Print and shaded views of the part. All mm, measured from the part's lowest x, y and z. Round coordinates to 2 decimals unless told otherwise and drop trailing zeros. Order: outer loops, then holes, each group sorted by start corner. A loop starts at its lowest first (then second) coordinate and runs counter-clockwise, first axis right, second up. Notation, with made-up numbers: (33, 35.5) - (46, 35.5) arc R20 cw to (46, 46.5) - close; hole circle Ø6 at (-34, 37). An arc over 180 degrees is marked (long way). Return JSON: item names as keys, results as strings. Group by question number.
Item 1: Probe probe 1 along Z at (x, y) = (2.25, 1); probe 2 along Z at (x, y) = (6.5, 6.75); probe 3 along X at (y, z) = (3.75, 46.5). List the from-to ranges inside material, lowest first.
Item 2: Saw through at A-A on z = 8.5. List the corners of the cut face in (x, y), and give its area (3 significant figures).
Item 3: Drop flat-ended pins along their axis: pin 1 (3 mm diameter, centred on y = 6, z = 15, fed in from +X); pin 2 (1.5 mm diameter, centred on x = 6.5, z = 34.5, fed in from -Y); pin 3 (4 mm diameter, centred on x = 7, z = 24, fed in from +Y). Give the stop position or say it passes through.
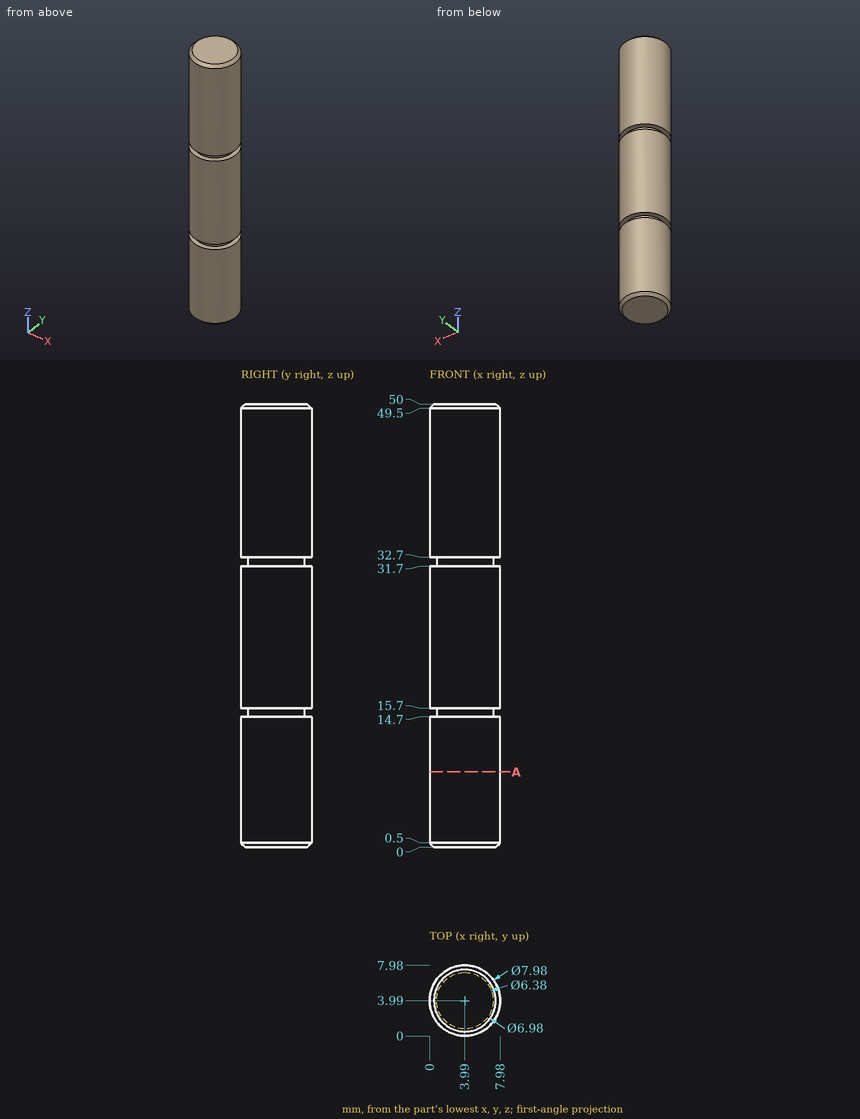
Filled in:
{
 "1": {"probe 1": "z = 0 to 14.7, 15.7 to 31.7, 32.7 to 50", "probe 2": "z = 0.24 to 14.7, 15.7 to 31.7, 32.7 to 49.76", "probe 3": "x = 0.01 to 7.97"},
 "2": {"outline": "circle Ø7.98 at (3.99, 3.99)", "area": "50.0 mm^2"},
 "3": {"pin 1": "stops at x = 7.94", "pin 2": "stops at y = 0.41", "pin 3": "stops at y = 7.85"}
}
